```python
from build123d import *

# Parameters (mm, degrees)
F1_DEPTH  = 7
F2_R      = 1.65
F3_DEPTH  = 25
F4_R      = 1.65
F5_DEPTH  = 25
F6_R      = 6.99999
F7_R      = 2.85
F8_DEPTH  = 1
F10_DEPTH = 1.5
F11_R     = 1.125
F13_R     = 1.125
F16_DEPTH = 25
F19_DEPTH = 1.1


# Not quite as in the source:
# - a fillet or chamfer is up to 0.001 mm smaller than in the source, because OpenCascade refuses the exact size
# - a feature names something its author has since deleted; it is built from what else it names


with BuildPart() as f1:
    # F0 (on Front) → F1 (new body, symmetric)
    with BuildSketch(Plane.XZ):
        Polygon((-39.5, 23.5411238112), (-39.5, 21.5411238112), (-39.5, -1.9508430529), (-35.5, -1.9508430529), (-35.5076822063, -3.4508233807), (-35.5076822063, -6.4508233807), (-29.5076822063, -6.4823476079), (-29.5076822063, -3.4823476079), (-29.5, -1.9823672801), (-25.5, -1.9823672801), (-25.5, 21.5411238112), (-25.5, 23.5411238112), (-29, 23.5411238112), (-29, 21.5334145057), (-29, 13.0334145057), (-36, 13.0334145057), (-36, 21.5411238112), (-36, 23.5411238112), align=None)
        Polygon((-29.5076822063, -6.4823476079), (-35.5076822063, -6.4508233807), (-35.5076822063, -13.9508233807), (-29.5076822063, -13.9508233807), align=None)
    extrude(amount=F1_DEPTH, both=True)

    # F2 (on face) → F3 (cut)
    with BuildSketch(Plane.YZ.offset(-29.5076822063)):
        with Locations((0, -10.2008233807)):
            Circle(F2_R)
    extrude(amount=-F3_DEPTH, mode=Mode.SUBTRACT)

    # F4 (on face) → F5 (cut)
    with BuildSketch(Plane.YZ.offset(-25.5)):
        with Locations((0, 17.2911238112)):
            Circle(F4_R)
    extrude(amount=-F5_DEPTH, mode=Mode.SUBTRACT)

    # F6 (radius 7 in the source; OpenCascade refuses exactly that, so slightly less here)
    f6_edges = [f1.edges().sort_by_distance(p)[0] for p in [
        (-37.75, -7, 23.541124),
        (-37.75, 7, 23.541124),
        (-27.25, 7, 23.541124),
        (-27.25, -7, 23.541124),
        (-32.507682, -7, -13.950823),
        (-32.507682, 7, -13.950823),
    ]]
    fillet(f6_edges, radius=F6_R)

    # F7 (on face) → F8 (cut)
    with BuildSketch(Plane.YZ.offset(-25.5)):
        with Locations((0, 17.2911238112)):
            Circle(F7_R)
    extrude(amount=-F8_DEPTH, mode=Mode.SUBTRACT)

    # F9 (on face) → F10 (cut)
    with BuildSketch(Plane(origin=(-39.5, 0, 0), x_dir=(0, -1, 0), z_dir=(-1, 0, 0))):
        Polygon((-0.0683087897, 14.1156973306), (2.7158456051, 15.6442534237), (2.7841543949, 18.8196799042), (0.0683087897, 20.4665502917), (-2.7158456051, 18.9379941986), (-2.7841543949, 15.7625677181), align=None)
    extrude(amount=-F10_DEPTH, mode=Mode.SUBTRACT)

    # F11 (on face) → F12 (revolve)
    with BuildSketch(Plane.XZ.offset(7)):
        with Locations((-35.5, 7.298982876)):
            Circle(F11_R)
    revolve(axis=Axis((-32.5, -7, 3.0412955625), (0, 0, -1)))

    # F13 (on face) → F14 (revolve)
    with BuildSketch(Plane(origin=(0, 7, 0), x_dir=(-1, 0, 0), z_dir=(0, 1, 0))):
        with Locations((29.6073952019, 7.2832577271)):
            Circle(F13_R)
    revolve(axis=Axis((-32.5, 7, 3.0412955625), (0, 0, -1)))

    # F15 (on face) → F16 (cut)
    with BuildSketch(Plane.XY.offset(13.0334145057)):
        Polygon((-25.5, -7), (-29, -7), (-36, -7), (-39.5, -7), (-39.5, -13.4261082858), (-25.5, -13.4261082858), align=None)
    extrude(amount=-F16_DEPTH, mode=Mode.SUBTRACT)

    # F18 (on offset) → F19 (cut, symmetric)
    with BuildSketch(Plane.YZ.offset(-32.5)):
        with BuildLine():
            ThreePointArc((-7, 9.0029031262), (-4.8, 4.7040660741), (-7, 0.4052290221))
            Line((-7, 0.4052290221), (-7, -2.1252823574))
            ThreePointArc((-7, -2.1252823574), (-2.6, 4.7040660741), (-7, 11.5334145057))
            Line((-7, 11.5334145057), (-7, 9.0029031262))
        make_face()
    extrude(amount=F19_DEPTH, both=True, mode=Mode.SUBTRACT)


solid = f1.part
```
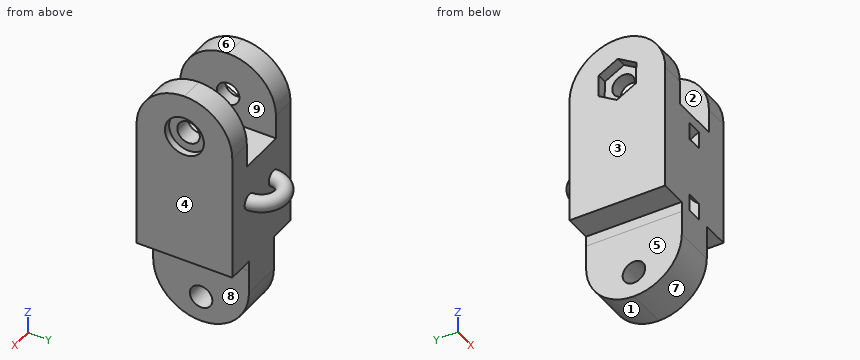
For this review, take the finished solid that the model builds, in its own axes (mm). Face numbers are marked on the shaded views. A direction names the side the tool comes from. Round coordinates to 2 decimals unless told otherwise and drop trailing zeros. Loops run counter-clockwise (first coordinate to the right, second up) from the corner with the lowest first, then second, coordinate; pieces in that order, holes last.
Q1. Add section B-B on z = 12.5. Write out the cut boundary in (x, y).
Result sheet:
outline: (-39.5, -7) - (-25.5, -7) - (-25.5, 7) - (-39.5, 7) - close
Q2. Machinability: for the marked faces 5, 6, 7, 8 and 9, which of the approach directions +Z, -Z, +X, -X, +Y, -Y give a long, thin tool a straight path to every point of the face, cutting with its end or side? Answer none if there is none.
Result sheet:
face 5: -Z, -X, +Y, -Y
face 6: +Z, +X, -X, -Y
face 7: -Z, +X, -X, -Y
face 8: -Z, +X, +Y, -Y
face 9: +Z, +Y, -Y
Q3. Add section A-A on z = 1. Write out the cut boundary in (x, y), plus the area to 3 significant figures.
Result sheet:
outline: (-39.5, -7) - (-25.5, -7) - (-25.5, 7) - (-39.5, 7) - close; hole (-33.6, -6.31) - (-31.4, -6.31) - (-31.4, -3.58) - (-33.6, -3.58) - close
area: 190 mm2
Q4. Insertion check: pin 1 Ø4 at (y, z) = (0, 17.29) entering from -X; pin 2 Ø8.5 at (y, z) = (-1, 18.5) entering from -X; pin 3 Ø5 at (y, z) = (0, -8) entering from -X; pin 4 Ø2 at (x, y) = (-33, 0) entering from +Z. Each pin has a flat end and moves straight along its axis. Give the tip position at first contact, or say it passes through.
Result sheet:
pin 1: stops at x = -38
pin 2: stops at x = -39.5
pin 3: stops at x = -35.51
pin 4: stops at z = 13.03
Q5. Mouldability with a two-part tool opening along X and no side actions: class the marked faces 1, 2, 3 and 4 as +X half, -X half, draft (parallel to the pull), parting line (faces both ways), or undercut.
Result sheet:
face 1: draft
face 2: undercut
face 3: -X half
face 4: +X half
Q6. To check wall thickness, follow line 1 along Z through (x, y) = (-27.7, 0); line 2 along Z through (x, y) = (-31.15, 0); line 3 along X through (y, z) = (-4.75, 2). State the ranges of each line that lie inside material, in increasing order.
Result sheet:
line 1: z = -1.98 to 15.64, 18.94 to 23.54
line 2: z = -13.95 to -11.85, -8.55 to 13.03
line 3: x = -39.5 to -33.6, -31.4 to -25.5
